from build123d import *

# Parameters (mm, degrees)
F1_DEPTH = 25
F3_D     = 5


with BuildPart() as f1:
    # F0 (on Front) → F1 (new body)
    with BuildSketch(Plane.XZ):
        Polygon((-122.5, 30), (-122.5, 0), (0, 0), (0, 70), (-75, 70), (-75, 30), align=None)
        Polygon((0, 70), (0, 0), (122.5, 0), (122.5, 30), (75, 30), (75, 70), align=None)
    extrude(amount=F1_DEPTH)

    # F3 (through all)
    with Locations(Plane.YZ.offset(122.5)):
        with Locations((-12.5, 15)):
            Hole(F3_D / 2)


solid = f1.part
Read the model definition and answer for the solid it produces. Units are mm, in the model's axes. A direction names the side the tool comes from. Coordinates: 2 decimals unless noted, no trailing zeros. Order: outer loops, then holes, each group sorted by start corner. A loop starts at its lowest first (then second) coordinate and runs counter-clockwise, first axis right, second up. Notation, with made-up numbers: (36, 7) -> (80, 7) arc R35 cw to (80, 39) -> close; hole circle Ø9 at (-20, 43.5). An arc over 180 degrees is marked (long way). Answer as a JSON object with one key per item and string values.
1) A cutting plane is placed at C-C, the plane x = -102.5. Determine the outline of the cut face in (y, z).
Model answer:
{"outline": "(-25, 0) -> (0, 0) -> (0, 30) -> (-25, 30) -> close; hole circle Ø5 at (-12.5, 15)"}
2) The mould has two halves that part along Z. Classify faces 1 (the face through (-2, -10, 15)), 2 (the face through (-2, 0, 28)), 3 (the face through (-98, -12, 30)): released by +Z, released by -Z, zero draft, split by the parting line, or undercut.
Model answer:
{"face 1": "undercut", "face 2": "zero draft", "face 3": "released by +Z"}
3) Each of these flat-tipped pins is pushed along its axis until it touches: pin 1 (7.5 mm diameter, centred on y = -8, z = 56, fed in from -X); pin 2 (5 mm diameter, centred on x = 97, y = -11.5, fed in from +Z); pin 3 (2 mm diameter, centred on y = -20, z = 34, fed in from +X). Where does it stop, or does it pass through?
Model answer:
{"pin 1": "stops at x = -75", "pin 2": "stops at z = 30", "pin 3": "stops at x = 75"}
4) Consider line 1 along Z through (x, y) = (8, -12.5); line 2 along Z through (x, y) = (77.5, -12.5); line 3 along Y through (x, z) = (73.5, 13). Determine where each line is inside the solid, lowest interval first. Write a range as from..to.
Model answer:
{"line 1": "z = 0..12.5, 17.5..70", "line 2": "z = 0..12.5, 17.5..30", "line 3": "y = -25..-14, -11..0"}
5) A tool of negligible diameter and unlimited length cuts with its end or side. For faces 4 (the face through (-75, -12, 50)), 5 (the face through (1, -12, 70)), 6 (the face through (75, -12, 50)), from which of +Z, -Z, +X, -X, +Y, -Y can it reach the whole face along a straight path? Write none if from no direction.
Model answer:
{"face 4": "+Z, -X, +Y, -Y", "face 5": "+Z, +X, -X, +Y, -Y", "face 6": "+Z, +X, +Y, -Y"}
6) A cutting plane is placed at A-A, the plane z = 15. Determine the outline of the cut face in (x, y).
Model answer:
{"outline": "(-122.5, -25) -> (122.5, -25) -> (122.5, -15) -> (-122.5, -15) -> close; (-122.5, -10) -> (122.5, -10) -> (122.5, 0) -> (-122.5, 0) -> close"}
7) A cutting plane is placed at B-B, the plane y = -12.5. Determine the outline of the cut face in (x, z), plus the area to 3 significant figures.
Model answer:
{"outline": "(-122.5, 0) -> (122.5, 0) -> (122.5, 12.5) -> (-122.5, 12.5) -> close; (-122.5, 17.5) -> (122.5, 17.5) -> (122.5, 30) -> (75, 30) -> (75, 70) -> (-75, 70) -> (-75, 30) -> (-122.5, 30) -> close", "area": "12,100 mm²"}
8) A cutting plane is placed at D-D, the plane z = 63.5. Determine the outline of the cut face in (x, y), plus the area to 3 significant figures.
Model answer:
{"outline": "(-75, -25) -> (75, -25) -> (75, 0) -> (-75, 0) -> close", "area": "3,750 mm²"}
